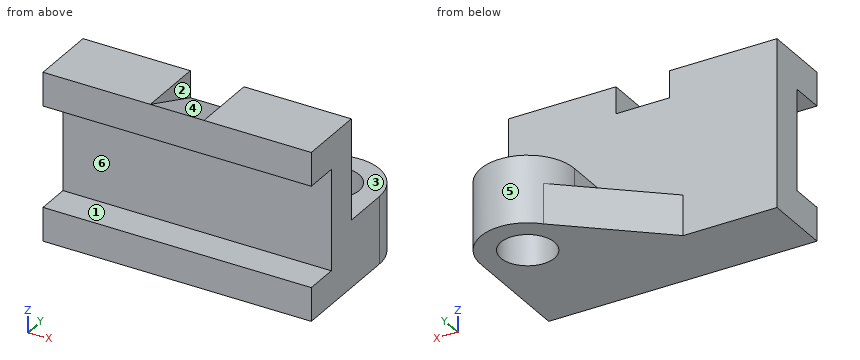
from build123d import *

# Parameters (mm, degrees)
SKETCH1_W           = 200
SKETCH1_H           = 125
BOSS_EXTRUDE2_DEPTH = 50
SKETCH3_R           = 20
BOSS_EXTRUDE5_DEPTH = 50
SKETCH6_W           = 75
SKETCH6_H           = 25
CUT_EXTRUDE1_DEPTH  = 242.466871434
BOSS_EXTRUDE6_DEPTH = 30
SKETCH8_W           = 40
SKETCH8_H           = 50
CUT_EXTRUDE2_DEPTH  = 20
BOSS_EXTRUDE7_DEPTH = 40


with BuildPart() as part:
    # Sketch1 → Boss-Extrude2 (new body)
    with BuildSketch(Plane(origin=(0, 0, 0), x_dir=(1, 0, 0), z_dir=(0, 1, 0))):
        Rectangle(SKETCH1_W, SKETCH1_H)
    extrude(amount=BOSS_EXTRUDE2_DEPTH)

    # Sketch3 → Boss-Extrude5 (add)
    with BuildSketch(Plane(origin=(0, 0, -62.5), x_dir=(-1, 0, 0), z_dir=(0, 0, -1))):
        with BuildLine():
            Line((-100, 50), (-100, 85))
            ThreePointArc((-100, 85), (-65, 120), (-30, 85))
            Line((-30, 85), (-30, 50))
            Line((-30, 50), (-100, 50))
        make_face()
        with Locations((-65, 85)):
            Circle(SKETCH3_R, mode=Mode.SUBTRACT)
    extrude(amount=-BOSS_EXTRUDE5_DEPTH)

    # Sketch6 → Cut-Extrude1 (cut, through all)
    with BuildSketch(Plane.ZY.offset(100)):
        with Locations((0, 12.5)):
            Rectangle(SKETCH6_W, SKETCH6_H)
    extrude(amount=-CUT_EXTRUDE1_DEPTH, mode=Mode.SUBTRACT)

    # Sketch7 → Boss-Extrude6 (add)
    with BuildSketch(Plane(origin=(0, 0, -62.5), x_dir=(-1, 0, 0), z_dir=(0, 0, -1))):
        with BuildLine():
            Line((-39.10827581, 108.550342215), (30, 50))
            Line((30, 50), (-30, 50))
            Line((-30, 50), (-30, 85))
            ThreePointArc((-30, 85), (-32.356391539, 97.625166402), (-39.10827581, 108.550342215))
        make_face()
    extrude(amount=-BOSS_EXTRUDE6_DEPTH)

    # Sketch8 → Cut-Extrude2 (cut)
    with BuildSketch(Plane.XY.offset(62.5)):
        with Locations((0, 25)):
            Rectangle(SKETCH8_W, SKETCH8_H)
    extrude(amount=-CUT_EXTRUDE2_DEPTH, mode=Mode.SUBTRACT)

    # Sketch9 → Boss-Extrude7 (add)
    with BuildSketch(Plane.ZY.offset(-20)):
        Polygon((42.5, 50), (62.5, 0), (42.5, 0), align=None)
    extrude(amount=BOSS_EXTRUDE7_DEPTH)


solid = part.part
Here's how the part is built. I have some questions about the finished solid (model axes, mm). Face numbers are marked on the shaded views. A direction names the side the tool comes from. Coordinates: 2 decimals unless noted, no trailing zeros. Order: outer loops, then holes, each group sorted by start corner. A loop starts at its lowest first (then second) coordinate and runs counter-clockwise, first axis right, second up. Notation, with made-up numbers: M 76.5,4.5 L 128.5,4.5 A22 cw 128.5,29.5 Z; hole C 51.5,74.25 d7. An arc over 180 degrees is marked long. Answer as CSV lines item,"result". Start each with the question number.
1. I want a section at A-A, the plane y = 13. Write out the boundary of the cut face in (x, z).
2. On a 3-axis mill with a long thin cutter (end or side, diameter ignored), from which of +Z, -Z, +X, -X, +Y, -Y can I reach the whole of each face in a straight line? I mean the marked faces 1, 2 and 3. Say none if no direction works.
3. I want a section at B-B, the plane x = 65. Write out the boundary of the cut face in (y, z), and give its area (4 significant figures).
4. I want a section at D-D, the plane z = 50. Write out the boundary of the cut face in (x, y).
5. For pin 1 (10 mm diameter, centred on x = 39, z = -26.5, fed in from +Y); pin 2 (1 mm diameter, centred on x = -48.5, z = 10, fed in from -Y); pin 3 (10 mm diameter, centred on x = 46, y = 66.5, fed in from +Z), each with a flat end and sliding along its axis, tell me the tip position at first contact or that it passes through.
6. I need wall thicknesses on line 1 (Y direction, x = 65, z = -47); line 2 (Z direction, x = -79, y = 16); line 3 (Y direction, x = 65, z = -31.5). Which ranges of each line are inside material? Lowest first, please. Write a range as [from, to].
7. We'd pull the mould along X, two halves only. Please class the marked faces 4, 5 and 6: released by +X, released by -X, zero draft, split by the parting line, or undercut.
8. I want a section at C-C, the plane z = -35. Write out the boundary of the cut face in (x, y).
Recorded:
1,outline,"M -100,-62.5 L 100,-62.5 L 100,-37.5 L -100,-37.5 Z; M -100,37.5 L 100,37.5 L 100,62.5 L 20,62.5 L 20,57.3 L -20,57.3 L -20,62.5 L -100,62.5 Z"
2,face 1,"+X, -X, -Y"
2,face 2,"+Z, +Y"
2,face 3,"+Z, +X, -X, +Y"
3,outline,"M 0,-62.5 L 65,-62.5 L 65,-12.5 L 50,-12.5 L 50,62.5 L 0,62.5 L 0,37.5 L 25,37.5 L 25,-37.5 L 0,-37.5 Z; M 105,-62.5 L 120,-62.5 L 120,-12.5 L 105,-12.5 Z"
3,area,"5,875 mm2"
4,outline,"M -100,0 L 100,0 L 100,50 L 20,50 L 20,31.25 L -20,31.25 L -20,50 L -100,50 Z"
5,pin 1,"stops at y = 113"
5,pin 2,"stops at y = 25"
5,pin 3,"stops at z = -12.5"
6,line 1,"y = [0, 65], [105, 120]"
6,line 2,"z = [-62.5, -37.5], [37.5, 62.5]"
6,line 3,"y = [25, 65], [105, 120]"
7,face 4,"undercut"
7,face 5,"split by the parting line"
7,face 6,"zero draft"
8,outline,"M -100,25 L 100,25 L 100,85 A35 ccw 39.11,108.55 L -30,50 L -100,50 Z; hole C 65,85 d40"
